Autodesk Inventor part; units mm, degrees
ref_plane "YZ Plane" through (0, 0, 0) normal (1, 0, 0) x (0, 1, 0)
ref_plane "XZ Plane" through (0, 0, 0) normal (0, 1, 0) x (-1, 0, 0)
ref_plane "XY Plane" through (0, 0, 0) normal (0, 0, 1) x (1, 0, 0)
sketch "Sketch1" plane through (0, 0, 0) normal (0, 0, 1) x (1, 0, 0)
  line L0 (-5, -2.5) -> (5, -2.5) construction
  line L1 (5, -2.5) -> (12.675, 0) construction
  line L2 (-5, -2.5) -> (-12.675, 0)
  line L3 (12.675, 0) -> (-12.675, 0) construction
  line L4 (12.675, 0) -> (12.675, 8.7) construction
  line L5 (-12.675, 0) -> (-12.675, 8.7)
  line L6 (-12.675, 8.7) -> (-4.75, 23.2)
  line L7 (-4.75, 23.2) -> (-4.75, 25.7)
  line L8 (-4.75, 25.7) -> (4.75, 25.7) construction
  line L9 (4.75, 25.7) -> (4.75, 23.2) construction
  line L10 (4.75, 23.2) -> (12.675, 8.7) construction
  line L11 (0, -8.56) -> (0, 31.76)
  line L12 (0, 25.7) -> (0, -2.5)
  circle A0 centre (-10.8, 4.25) radius 1.25
  line L13 (-10.8, 4.25) -> (0, 4.25) construction
  line L14 (-4.75, 25.7) -> (0, 25.7)
  line L15 (-5, -2.5) -> (0, -2.5)
  line L16 (-5.05, 23.2766) -> (-12.975, 8.7766)
  line L17 (-12.975, 8.7766) -> (-12.975, -0.2178)
  line L18 (-12.975, -0.2178) -> (-5.0476, -2.8)
  line L19 (-5.0476, -2.8) -> (0.3, -2.8) construction
  line L20 (0.3, -2.8) -> (0.3, 26) construction
  line L21 (0.3, 26) -> (-5.05, 26) construction
  line L22 (-5.05, 26) -> (-5.05, 23.2766)
  line L23 (0, -2.5) -> (0, -2.8)
  line L24 (0, 25.7) -> (0, 26)
  line L25 (0, -2.8) -> (-5.0476, -2.8)
  line L26 (0, 26) -> (-5.05, 26)
  point P0 (0, 0)
  point P1 (0, 0)
  dimension "d0" = 10
  dimension "d1" = 25.35
  dimension "d2" = 2.5
  dimension "d3" = 8.7
  dimension "d4" = 28.2
  dimension "d6" = 2.5
  dimension "d7" = 9.5
  dimension "d42" = 2.5
  dimension "d43" = 10.8
  dimension "d44" = 6.75
  dimension "d53" = 0.3
sketch "Sketch8" plane through (0, 0, 0) normal (0, 0, 1) x (1, 0, 0)
  line L0 (-20, 30) -> (20, 30)
  line L1 (20, 30) -> (20, -10)
  line L2 (20, -10) -> (-20, -10)
  line L3 (-20, -10) -> (-20, 30)
  point P0 (0, 0)
  point P1 (0, -10)
  dimension "d45" = 40
  dimension "d46" = 10
extrude "MainBlock" add sketch "Sketch8" against normal blind 7
extrude "CartridgeCutout" cut sketch "Sketch1" against normal blind 3
sketch "Sketch10" plane through (-10.8, 4.25, 0) normal (0, 0, 1) x (1, 0, 0)
  circle A0 centre (0, 0) radius 1.25
  circle A1 centre (0, 0) radius 1.45
  point P0 (10.8, -4.25)
  dimension "d56" = 0.2
extrude "PinHole" cut sketch "Sketch10" against normal through all contours A0 | A1
mirror "Mirror3" about plane through (0, 26, 0) normal (-1, 0, 0) of "CartridgeCutout", "PinHole"
sketch "Sketch12" plane through (0, 0, -3) normal (0, 0, 1) x (1, 0, 0)
  circle A0 centre (10.8, 4.25) radius 1.45
  circle A1 centre (-10.8, 4.25) radius 1.45
  line L0 (5.05, 26) -> (-5.05, 26)
  line L1 (-5.05, 23.2766) -> (-5.05, 26)
  line L2 (-12.975, 8.7766) -> (-5.05, 23.2766)
  line L3 (-12.975, -0.2178) -> (-12.975, 8.7766)
  line L4 (-5.0476, -2.8) -> (-12.975, -0.2178)
  line L5 (5.0476, -2.8) -> (-5.0476, -2.8)
  line L6 (5.0476, -2.8) -> (12.975, -0.2178)
  line L7 (12.975, -0.2178) -> (12.975, 8.7766)
  line L8 (12.975, 8.7766) -> (5.05, 23.2766)
  line L9 (5.05, 23.2766) -> (5.05, 26)
  line L10 (-4.15, 23.6) -> (4.15, 23.6)
  line L11 (4.15, 23.6) -> (4.15, -1.4)
  line L12 (4.15, -1.4) -> (-4.15, -1.4)
  line L13 (-4.15, -1.4) -> (-4.15, 23.6)
  point P0 (0, 0)
  point P1 (0, -1.4)
  dimension "d59" = 8.3
  dimension "d60" = 25
  dimension "d61" = 1.4
extrude "CentreHole" cut sketch "Sketch12" against normal through all contours L10 L11 L12 L13
sketch "Sketch13" plane through (0, 0, 0) normal (0, 0, 1) x (1, 0, 0)
  line L0 (-5.05, 26) -> (5.05, 26)
  line L1 (5.05, 26) -> (5.05, 23.2766)
  line L2 (5.05, 23.2766) -> (12.975, 8.7766)
  line L3 (12.975, 8.7766) -> (12.975, -0.2178)
  line L4 (12.975, -0.2178) -> (5.0476, -2.8)
  line L5 (5.0476, -2.8) -> (-5.0476, -2.8)
  line L6 (-5.0476, -2.8) -> (-12.975, -0.2178)
  line L7 (-12.975, -0.2178) -> (-12.975, 8.7766)
  line L8 (-12.975, 8.7766) -> (-5.05, 23.2766)
  line L9 (-5.05, 23.2766) -> (-5.05, 26)
  line L10 (-20, 30) -> (20, 30)
  line L11 (-20, -10) -> (-20, 30)
  line L12 (20, -10) -> (-20, -10)
  line L13 (20, 30) -> (20, -10)
  line L14 (-14.975, 9.2875) -> (-14.975, -1.6698)
  line L15 (-14.975, -1.6698) -> (-5.3652, -4.8)
  line L16 (-5.3652, -4.8) -> (5.3652, -4.8)
  line L17 (5.3652, -4.8) -> (14.975, -1.6698)
  line L18 (14.975, -1.6698) -> (14.975, 9.2875)
  line L19 (14.975, 9.2875) -> (7.05, 23.7875)
  line L20 (7.05, 23.7875) -> (7.05, 28)
  line L21 (7.05, 28) -> (-7.05, 28)
  line L22 (-7.05, 28) -> (-7.05, 23.7875)
  line L23 (-7.05, 23.7875) -> (-14.975, 9.2875)
  point P0 (0, 0)
  dimension "d65" = 2
extrude "OutlineCut" cut sketch "Sketch13" against normal through all contours L10 L13 L12 L11
sketch "Sketch14" plane through (0, 0, -3) normal (0, 0, 1) x (1, 0, 0)
  line L0 (-4.15, -1.4) -> (-4.15, 23.6)
  line L1 (-4.15, 23.6) -> (4.15, 23.6)
  line L2 (4.15, 23.6) -> (4.15, -1.4)
  line L3 (4.15, -1.4) -> (-4.15, -1.4) construction
  circle A0 centre (10.8, 4.25) radius 1.45 construction
  circle A1 centre (-10.8, 4.25) radius 1.45 construction
  line L4 (5.05, 26) -> (-5.05, 26)
  line L5 (-5.05, 23.2766) -> (-5.05, 26)
  line L6 (-12.975, 8.7766) -> (-5.05, 23.2766)
  line L7 (-12.975, -0.2178) -> (-12.975, 8.7766) construction
  line L8 (-5.0476, -2.8) -> (-12.975, -0.2178) construction
  line L9 (5.0476, -2.8) -> (-5.0476, -2.8) construction
  line L10 (5.0476, -2.8) -> (12.975, -0.2178) construction
  line L11 (12.975, -0.2178) -> (12.975, 8.7766) construction
  line L12 (12.975, 8.7766) -> (5.05, 23.2766)
  line L13 (5.05, 23.2766) -> (5.05, 26)
  line L14 (-9.7922, 14.6) -> (-4.15, 14.6)
  line L15 (-12.975, 8.7766) -> (-5.05, 23.2766)
  line L16 (-4.15, 23.6) -> (-5.05, 23.2766)
  line L17 (0, -18) -> (0, 38)
  line L18 (-4.15, 23.6) -> (-4.15, 14.6)
  line L19 (-4.15, -1.4) -> (-4.15, 23.6)
  line L20 (-5.05, 23.2766) -> (-9.7922, 14.6)
  line L21 (-12.975, 8.7766) -> (-5.05, 23.2766)
  line L22 (9.7922, 14.6) -> (4.15, 14.6)
  line L23 (4.15, 23.6) -> (5.05, 23.2766)
  line L24 (4.15, 23.6) -> (4.15, 14.6)
  line L25 (5.05, 23.2766) -> (9.7922, 14.6)
  point P0 (0, 0)
  dimension "d70" = 9
extrude "AlignmentGooveCut" cut sketch "Sketch14" against normal blind 1 contours L14 L6 L16 L0 | L23 L12 L22 L2
sketch "Sketch16" plane through (0, 0, 0) normal (0, 0, 1) x (1, 0, 0)
  line L0 (-8.5, 12.6) -> (8.5, 12.6)
  line L1 (8.5, 12.6) -> (8.5, -7.4)
  line L2 (8.5, -7.4) -> (-8.5, -7.4)
  line L3 (-8.5, -7.4) -> (-8.5, 12.6)
  line L4 (4.15, -1.4) -> (-4.15, -1.4)
  point P0 (0, 0)
  point P1 (0, -7.4)
  dimension "d73" = 17
  dimension "d74" = 20
  dimension "d75" = 14
extrude "CircuitBoardCut" cut sketch "Sketch16" against normal blind 6
sketch "Sketch18" plane through (0, 0, -6) normal (0, 0, 1) x (1, 0, 0)
  line L0 (-4.15, 12.6) -> (-4.15, -1.4)
  line L1 (-4.15, -1.4) -> (4.15, -1.4)
  line L2 (4.15, -1.4) -> (4.15, 12.6)
  line L3 (-4.15, 12.6) -> (4.15, 12.6)
  line L4 (-4.15, 23.6) -> (-4.15, -1.4)
  point P0 (0, 0)
extrude "CircuitBoardFillIn" add sketch "Sketch18" against normal up to surface (1 mm away)
sketch "Sketch19" plane through (0, 0, 0) normal (0, 0, 1) x (1, 0, 0)
  line L0 (8.5, -1.6754) -> (8.5, -3.7789)
  line L1 (8.5, -3.7789) -> (14.975, -1.6698)
  line L2 (14.975, -1.6698) -> (14.975, 9.2875)
  line L3 (14.975, 9.2875) -> (7.05, 23.7875)
  line L4 (7.05, 23.7875) -> (7.05, 28)
  line L5 (-7.05, 28) -> (-7.05, 23.7875)
  line L6 (-7.05, 23.7875) -> (-14.975, 9.2875)
  line L7 (-14.975, 9.2875) -> (-14.975, -1.6698)
  line L8 (-14.975, -1.6698) -> (-8.5, -3.7789)
  line L9 (-8.5, -3.7789) -> (-8.5, -1.6754)
  line L10 (-8.5, -1.6754) -> (-12.975, -0.2178)
  line L11 (-12.975, -0.2178) -> (-12.975, 8.7766)
  line L12 (-12.975, 8.7766) -> (-5.05, 23.2766)
  line L13 (-5.05, 23.2766) -> (-5.05, 26)
  line L14 (-5.05, 26) -> (5.05, 26)
  line L15 (5.05, 26) -> (5.05, 23.2766)
  line L16 (5.05, 23.2766) -> (12.975, 8.7766)
  line L17 (12.975, 8.7766) -> (12.975, -0.2178)
  line L18 (12.975, -0.2178) -> (8.5, -1.6754)
  line L19 (7.05, 28) -> (-7.05, 28)
  point P0 (0, 0)
extrude "TopHeightAdjustment" add sketch "Sketch19" along normal blind 0.3
sketch "Sketch20" plane through (0, 0, 0.3) normal (0, 0, 1) x (1, 0, 0)
  line L0 (-20, -14.6) -> (20, -14.6)
  line L1 (20, -14.6) -> (20, 14.6)
  line L2 (20, 14.6) -> (-20, 14.6)
  line L3 (-20, 14.6) -> (-20, -14.6)
  line L4 (-4.15, 14.6) -> (-9.7922, 14.6)
  point P0 (0, 0)
  point P1 (0, 14.6)
  point P2 (-20, 0)
  dimension "d89" = 40
extrude "Extrusion19" cut sketch "Sketch20" against normal through all
sketch "Sketch21" plane through (0, 0, 0.3) normal (0, 0, 1) x (1, 0, 0)
  line L0 (-12.0715, 14.6) -> (-9.7922, 14.6)
  line L1 (-9.7922, 14.6) -> (-5.05, 23.2766)
  line L2 (-5.05, 23.2766) -> (-5.05, 26)
  line L3 (-5.05, 26) -> (5.05, 26)
  line L4 (5.05, 26) -> (5.05, 23.2766)
  line L5 (5.05, 23.2766) -> (9.7922, 14.6)
  line L6 (9.7922, 14.6) -> (12.0715, 14.6)
  line L7 (12.0715, 14.6) -> (7.05, 23.7875)
  line L8 (7.05, 23.7875) -> (7.05, 28)
  line L9 (7.05, 28) -> (-7.05, 28)
  line L10 (-7.05, 28) -> (-7.05, 23.7875)
  line L11 (-7.05, 23.7875) -> (-12.0715, 14.6)
  point P0 (0, 0)
extrude "Extrusion20" add sketch "Sketch21" along normal blind 3
fillet "Fillet4" radius 1 6 edges at (-12.0715, 14.6, -1.85) (12.0715, 14.6, -1.85) (7.05, 28, -1.85) (4.15, 14.6, -5.5) (-4.15, 14.6, -5.5) (-7.05, 28, -1.85)
properties part number "TestShroud"
Source: CAD feature listing. Evaluate the final solid. Frame: model axes, mm. A direction names the side the tool comes from. Give positions to 0.01 mm unless a question says otherwise; leave off trailing zeros. Loops run counter-clockwise (first coordinate to the right, second up) from the corner with the lowest first, then second, coordinate; pieces in that order, holes last. Notation, with made-up numbers: (-6, 83.5) -> (3, 83.5) arc R23 cw to (3, 95.5) -> close; hole circle Ø4 at (-30, 82). An arc over 180 degrees is marked (long way). Put each result on its own line as item: value. Start each with the question number.
1) Material intervals for probe 1 along X at (y, z) = (25.5, 2); probe 2 along Y at (x, z) = (-3, -2); probe 3 along Y at (x, z) = (1.25, -5.75), sorted ascending.
2) Contact query for flat-ended pins moving along their axis: P1, Ø0.8, axis at y = 24.5, z = -1, coming from the -X side; P2, Ø5, axis at x = -0.5, y = 16.5, coming from the +Z side; P3, Ø0.9, axis at y = 20.5, z = -5, coming from the +X side; P4, Ø4, axis at y = 20.5, z = -4.5, coming from the +X side. Output: stop coordinate, or through.
3) Reachability of faces 1 (the face through (-6, 18, -4)), 2 (the face through (-7.05, 25, -2)), 3 (the face through (4.451, 14.885, -5.521)) from +Z, -Z, +X, -X, +Y, -Y: full face, straight path, thin tool, end or side. Return the list, or none.
4) Cut plane D-D (y = 25). Return loops of the section in (x, z).
5) Cut plane A-A (z = -0.5). Return loops of the section in (x, y).
6) Cut plane C-C (x = 9). Return loops of the section in (y, z), then the cut area to 3 significant figures.
7) Cut plane B-B (y = 19). Return loops of the section in (x, z), then the cut area to 3 significant figures.
Results are:
1. probe 1: x = -7.05 to -5.05, 5.05 to 7.05
1. probe 2: y = 26 to 28
1. probe 3: y = 23.6 to 28
2. P1: stops at x = -7.05
2. P2: passes through
2. P3: stops at x = 9.09
2. P4: stops at x = 9.94
3. face 1: +Z, -Y
3. face 2: +Z, -Z, -X, +Y
3. face 3: +Z, -Z, -Y
4. outline: (-7.05, -7) -> (7.05, -7) -> (7.05, 3.3) -> (5.05, 3.3) -> (5.05, -3) -> (-5.05, -3) -> (-5.05, 3.3) -> (-7.05, 3.3) -> close
5. outline: (-11.26, 16.08) arc R1 ccw to (-10.39, 14.6) -> (-9.79, 14.6) -> (-5.05, 23.28) -> (-5.05, 26) -> (5.05, 26) -> (5.05, 23.28) -> (9.79, 14.6) -> (10.39, 14.6) arc R1 ccw to (11.26, 16.08) -> (7.05, 23.79) -> (7.05, 27) arc R1 ccw to (6.05, 28) -> (-6.05, 28) arc R1 ccw to (-7.05, 27) -> (-7.05, 23.79) -> close
6. outline: (14.6, -7) -> (20.22, -7) -> (20.22, 3.3) -> (16.05, 3.3) -> (16.05, -4) -> (14.6, -4) -> close
6. area: 47.3 mm2
7. outline: (-9.67, -7) -> (-4.15, -7) -> (-4.15, -4) -> (-7.39, -4) -> (-7.39, 3.3) -> (-9.67, 3.3) -> close; (4.15, -7) -> (9.67, -7) -> (9.67, 3.3) -> (7.39, 3.3) -> (7.39, -4) -> (4.15, -4) -> close
7. area: 66.4 mm2
